Source: CAD feature listing. Evaluate the final solid. Frame: model axes, mm. Face numbers are marked on the shaded views. Round coordinates to 2 decimals unless told otherwise and drop trailing zeros. Loops run counter-clockwise (first coordinate to the right, second up) from the corner with the lowest first, then second, coordinate; pieces in that order, holes last.
Item 1: Ray query, L1, parallel to X at y = 1.15, z = 0; L2, parallel to Y at x = 12.75, z = 1; L3, parallel to Z at x = 5, y = 2.6. Return the intervals inside material, ascending.
Item 2: Section query B-B on x = 2. Return loops of the section in (y, z).
Item 3: Section query A-A on z = 0. Return loops of the section in (x, y), then the cut area to 3 significant figures.
Item 4: Section query D-D on x = 9. Return loops of the section in (y, z), then the cut area to 3 significant figures.
Item 5: Section query C-C on y = 0.6. Return loops of the section in (x, z) (3 decimals), then the cut area to 3 significant figures.
Item 6: Pull-direction query (Z, two-part tool) for the marked faces 1, 2 and 3; classes: released by +Z, released by -Z, zero draft, split by the parting line, or undercut.
Item 7: First-contact query: P1, Ø1, axis at x = 2, z = 1, coming from the +Y side; P2, Ø1.5, axis at x = -3, y = 2.5, coming from the -Z side; P3, Ø5.5, axis at x = 6.5, z = 1, coming from the +Y side. Flat tips, straight axial feed; report the tip coordinate or a pass-through.
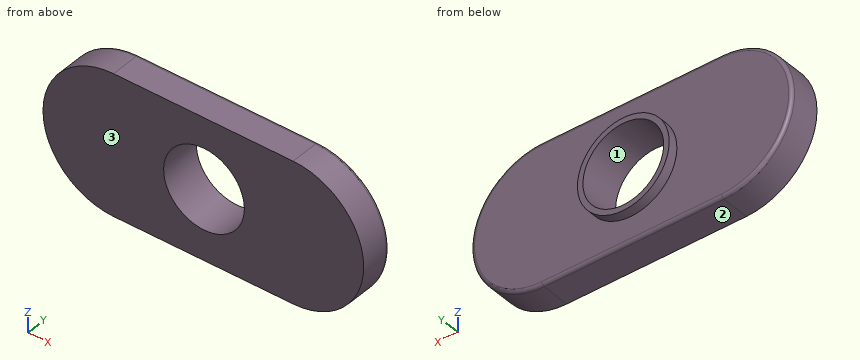
```python
from build123d import *

# Parameters (mm, degrees)
BOSS_EXTRUDE1_DEPTH = 2.4638
SKETCH2_R           = 3.6068
BOSS_EXTRUDE3_DEPTH = 0.762
SKETCH5_R           = 3.175
CUT_EXTRUDE2_DEPTH  = 21.693152562
FILLET1_R           = 0.254


with BuildPart() as part:
    # Sketch1 → Boss-Extrude1 (new body)
    with BuildSketch(Plane(origin=(0, 0, 0), x_dir=(1, 0, 0), z_dir=(0, 1, 0))):
        with BuildLine():
            Line((0, 5.5499), (14.1224, 5.5499))
            ThreePointArc((14.1224, 5.5499), (19.6723, 0), (14.1224, -5.5499))
            Line((14.1224, -5.5499), (0, -5.5499))
            ThreePointArc((0, -5.5499), (-5.5499, 0), (0, 5.5499))
        make_face()
    extrude(amount=BOSS_EXTRUDE1_DEPTH)

    # Sketch2 → Boss-Extrude3 (add)
    with BuildSketch(Plane(origin=(0, 2.4638, 0), x_dir=(1, 0, 0), z_dir=(0, 1, 0))):
        with Locations(Location((7.112, 0, 0), (0, 0, 90))):
            Circle(SKETCH2_R)
    extrude(amount=BOSS_EXTRUDE3_DEPTH)

    # Sketch5 → Cut-Extrude2 (cut, through all)
    with BuildSketch(Plane(origin=(0, 3.2258, 0), x_dir=(1, 0, 0), z_dir=(0, 1, 0))):
        with Locations(Location((7.112, 0, 0), (0, 0, 270))):
            Circle(SKETCH5_R)
    extrude(amount=-CUT_EXTRUDE2_DEPTH, mode=Mode.SUBTRACT)

    # Fillet1
    fillet1_edges = [part.edges().sort_by_distance(p)[0] for p in [
        (19.6723, 2.4638, 0),
        (7.0612, 2.4638, -5.5499),
        (-5.5499, 2.4638, 0),
        (7.0612, 2.4638, 5.5499),
    ]]
    fillet(fillet1_edges, radius=FILLET1_R)


solid = part.part
```
Data:
1. L1: x = -5.55 to 3.94, 10.29 to 19.67
1. L2: y = 0 to 2.46
1. L3: z = -2.92 to -2.37, 2.37 to 2.92
2. outline: (0, -5.55) - (2.21, -5.55) arc R0.25 ccw to (2.46, -5.3) - (2.46, 5.3) arc R0.25 ccw to (2.21, 5.55) - (0, 5.55) - close
3. outline: (-5.55, 0) - (3.94, 0) - (3.94, 3.23) - (3.51, 3.23) - (3.51, 2.46) - (-5.3, 2.46) arc R0.25 ccw to (-5.55, 2.21) - close; (10.29, 0) - (19.67, 0) - (19.67, 2.21) arc R0.25 ccw to (19.42, 2.46) - (10.72, 2.46) - (10.72, 3.23) - (10.29, 3.23) - close
3. area: 47.1 mm2
4. outline: (0, -5.55) - (2.21, -5.55) arc R0.25 ccw to (2.46, -5.3) - (2.46, -3.07) - (3.23, -3.07) - (3.23, -2.55) - (0, -2.55) - close; (0, 2.55) - (3.23, 2.55) - (3.23, 3.07) - (2.46, 3.07) - (2.46, 5.3) arc R0.25 ccw to (2.21, 5.55) - (0, 5.55) - close
4. area: 15.5 mm2
5. outline: (0, -5.55) - (14.122, -5.55) arc R5.55 ccw to (14.122, 5.55) - (0, 5.55) arc R5.55 ccw to start; hole circle Ø6.35 at (7.112, 0)
5. area: 222 mm2
6. face 1: undercut
6. face 2: released by -Z
6. face 3: zero draft
7. P1: stops at y = 2.46
7. P2: stops at z = -5.05
7. P3: stops at y = 3.23
